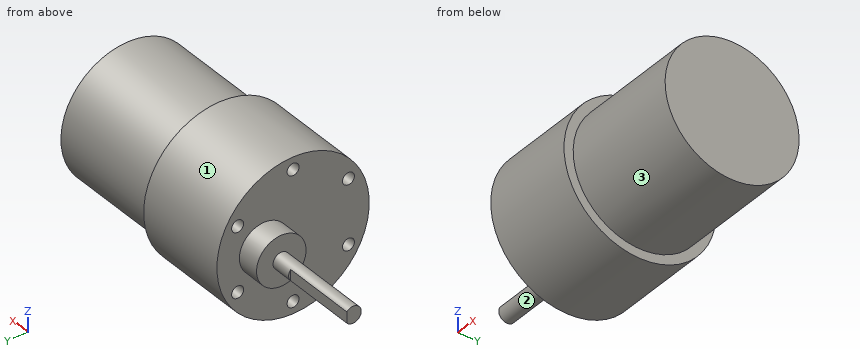
from build123d import *

# Parameters (mm, degrees)
SKETCH1_W                   = 23.5
SKETCH1_H                   = 18.45
SKETCH1_W_2                 = 29.5
SKETCH1_H_2                 = 16.23
M3_5X0_6_TAPPED_HOLE1_D     = 2.9
M3_5X0_6_TAPPED_HOLE1_DEPTH = 3.5
M3_5X0_6_TAPPED_HOLE1_TIP   = 0.871247898
SKETCH6_R                   = 6
BOSS_EXTRUDE1_DEPTH         = 5.5
SKETCH7_R                   = 2
BOSS_EXTRUDE2_DEPTH         = 23
CUT_EXTRUDE1_DEPTH          = 18


with BuildPart() as part:
    # Sketch1 → Revolve1 (revolve)
    with BuildSketch(Plane.XY, mode=Mode.PRIVATE) as revolve1_sk:
        with Locations((11.75, 9.225)):
            Rectangle(SKETCH1_W, SKETCH1_H)
        with Locations((38.25, 8.115)):
            Rectangle(SKETCH1_W_2, SKETCH1_H_2)
    revolve(revolve1_sk.sketch.rotate(Axis((0, 0, 0), (1, 0, 0)), 90), axis=Axis((0, 0, 0), (1, 0, 0)))

    # M3.5x0.6 Tapped Hole1
    with Locations(Plane.ZY):
        with Locations((7.75, 13.423393759), (15.5, 0), (7.75, -13.423393759), (-7.75, -13.423393759), (-15.5, 0), (-7.75, 13.423393759)):
            Hole(M3_5X0_6_TAPPED_HOLE1_D / 2, depth=M3_5X0_6_TAPPED_HOLE1_DEPTH)
            with Locations((0, 0, -(M3_5X0_6_TAPPED_HOLE1_DEPTH + M3_5X0_6_TAPPED_HOLE1_TIP / 2))):  # 118° drill point
                Cone(0, M3_5X0_6_TAPPED_HOLE1_D / 2, M3_5X0_6_TAPPED_HOLE1_TIP, mode=Mode.SUBTRACT)

    # Sketch6 → Boss-Extrude1 (add)
    with BuildSketch(Plane.ZY):
        with Locations((0, 7)):
            Circle(SKETCH6_R)
    extrude(amount=BOSS_EXTRUDE1_DEPTH)

    # Sketch7 → Boss-Extrude2 (add)
    with BuildSketch(Plane.ZY.offset(5.5)):
        with Locations((0, 7)):
            Circle(SKETCH7_R)
    extrude(amount=BOSS_EXTRUDE2_DEPTH)

    # Sketch8 → Cut-Extrude1 (cut)
    with BuildSketch(Plane.ZY.offset(28.5)):
        Polygon((-78.17402708, 8.5), (-1.322875656, 8.5), (1.322875656, 8.5), (78.17402708, 8.5), (78.17402708, 162.202302849), (-78.17402708, 162.202302849), align=None)
    extrude(amount=-CUT_EXTRUDE1_DEPTH, mode=Mode.SUBTRACT)


solid = part.part
For this review, take the finished solid that the model builds, in its own axes (mm). Face numbers are marked on the shaded views. A direction names the side the tool comes from. Give positions to 0.01 mm unless a question says otherwise; leave off trailing zeros. Loops run counter-clockwise (first coordinate to the right, second up) from the corner with the lowest first, then second, coordinate; pieces in that order, holes last.
Item 1: Take a section at A-A, the plane z = 0. State the section outline as (x, y) points.
Item 2: Take a section at D-D, the plane x = -17. State the section outline as (y, z) points, and give its area (3 significant figures).
Item 3: Insertion check: pin 1 (1.7 mm diameter, centred on y = -13.42, z = -7.75, fed in from -X); pin 2 (2.5 mm diameter, centred on y = 0, z = 15.5, fed in from -X); pin 3 (1.5 mm diameter, centred on x = 18, z = -1, fed in from +Y). Each pin has a flat end and moves straight along its axis. Give the tip position at first contact, or say it passes through.
Item 4: Take a section at C-C, the plane y = 7. State the section outline as (x, z) points.
Item 5: Tool access review of the marked faces 1, 2 and 3: name each direction out of +Z, -Z, +X, -X, +Y, -Y from which nothing blocks a thin tool from reaching the whole face with its end or side.
Item 6: For line 1 along Y through (x, z) = (1.5, -7.75); line 2 along Y through (x, z) = (1, 7); line 3 along X through (y, z) = (-5, -16), list the stretches that pass through material, from the lowest coordinate up.
Item 7: Take a section at B-B, the plane x = 19.5. State the section outline as (y, z) points, and give its area (3 significant figures).
Calculated:
1. outline: (-28.5, 5) - (-5.5, 5) - (-5.5, 1) - (0, 1) - (0, -18.45) - (23.5, -18.45) - (23.5, -16.23) - (53, -16.23) - (53, 16.23) - (23.5, 16.23) - (23.5, 18.45) - (0, 18.45) - (0, 13) - (-5.5, 13) - (-5.5, 9) - (-10.5, 9) - (-10.5, 8.5) - (-28.5, 8.5) - close
2. outline: (8.5, -1.32) - (8.5, 1.32) arc R2 ccw (long way) to start
2. area: 11.7 mm2
3. pin 1: stops at x = 3.86
3. pin 2: stops at x = 3.62
3. pin 3: stops at y = 18.45
4. outline: (-28.5, -2) - (-5.5, -2) - (-5.5, -6) - (0, -6) - (0, -17.07) - (23.5, -17.07) - (23.5, -14.64) - (53, -14.64) - (53, 14.64) - (23.5, 14.64) - (23.5, 17.07) - (0, 17.07) - (0, 6) - (-5.5, 6) - (-5.5, 2) - (-28.5, 2) - close
5. face 1: +X, -X
5. face 2: -X
5. face 3: +X
6. line 1: y = -16.74 to -14.87, -11.97 to 11.97, 14.87 to 16.74
6. line 2: y = -17.07 to -14.66, -12.18 to 12.18, 14.66 to 17.07
6. line 3: x = 0 to 23.5
7. outline: circle Ø36.9 at (0, 0)
7. area: 1,070 mm2
